from build123d import *

# Parameters (mm, degrees)
F1_DEPTH = 5
F2_R     = 1.5
F3_DEPTH = 25


with BuildPart() as f1:
    # F0 (on Front) → F1 (new body)
    with BuildSketch(Plane.XZ):
        with BuildLine():
            Line((-23, 75), (-27, 75))
            ThreePointArc((-27, 75), (-29.12132, 74.12132), (-30, 72))
            Line((-30, 72), (-30, -72))
            ThreePointArc((-30, -72), (-29.12132, -74.12132), (-27, -75))
            Line((-27, -75), (-23, -75))
            ThreePointArc((-23, -75), (-20.87868, -74.12132), (-20, -72))
            Line((-20, -72), (-20, -15))
            ThreePointArc((-20, -15), (-18.535534, -11.464466), (-15, -10))
            Line((-15, -10), (15, -10))
            ThreePointArc((15, -10), (18.535534, -11.464466), (20, -15))
            Line((20, -15), (20, -72))
            ThreePointArc((20, -72), (20.87868, -74.12132), (23, -75))
            Line((23, -75), (27, -75))
            ThreePointArc((27, -75), (29.12132, -74.12132), (30, -72))
            Line((30, -72), (30, 72))
            ThreePointArc((30, 72), (29.12132, 74.12132), (27, 75))
            Line((27, 75), (23, 75))
            ThreePointArc((23, 75), (20.87868, 74.12132), (20, 72))
            Line((20, 72), (20, 15))
            ThreePointArc((20, 15), (18.535534, 11.464466), (15, 10))
            Line((15, 10), (-15, 10))
            ThreePointArc((-15, 10), (-18.535534, 11.464466), (-20, 15))
            Line((-20, 15), (-20, 72))
            ThreePointArc((-20, 72), (-20.87868, 74.12132), (-23, 75))
        make_face()
        with BuildLine():
            Line((-23.600001, -71.399999), (-26.399999, -71.399999))
            Line((-26.399999, -71.399999), (-26.399999, 71.399999))
            Line((-26.399999, 71.399999), (-23.600001, 71.399999))
            Line((-23.600001, 71.399999), (-23.600001, 15))
            ThreePointArc((-23.600001, 15), (-21.081119, 8.918881), (-15, 6.399999))
            Line((-15, 6.399999), (15, 6.399999))
            ThreePointArc((15, 6.399999), (21.081119, 8.918881), (23.600001, 15))
            Line((23.600001, 15), (23.600001, 71.399999))
            Line((23.600001, 71.399999), (26.399999, 71.399999))
            Line((26.399999, 71.399999), (26.399999, -71.399999))
            Line((26.399999, -71.399999), (23.600001, -71.399999))
            Line((23.600001, -71.399999), (23.600001, -15))
            ThreePointArc((23.600001, -15), (21.081119, -8.918881), (15, -6.399999))
            Line((15, -6.399999), (-15, -6.399999))
            ThreePointArc((-15, -6.399999), (-21.081119, -8.918881), (-23.600001, -15))
            Line((-23.600001, -15), (-23.600001, -71.399999))
        make_face(mode=Mode.SUBTRACT)
    extrude(amount=F1_DEPTH)

    # F2 (on face) → F3 (cut)
    with BuildSketch(Plane.XY.offset(10)):
        with Locations((0, -2.50134)):
            Circle(F2_R)
    extrude(amount=-F3_DEPTH, mode=Mode.SUBTRACT)


solid = f1.part
CAD build for the part. Positions are in the model's coordinates, mm. A direction names the side the tool comes from. Coordinates: 2 decimals unless noted, no trailing zeros. Write each loop counter-clockwise with the first axis right and the second up, starting at its lowest first coordinate (ties: lowest second). Pieces come first, ordered by that corner, then holes. Notation, with made-up numbers: (87, 75) - (119, 75) arc R34 cw to (119, 111) - close; hole circle Ø2 at (47, 48). An arc over 180 degrees is marked (long way). Use a Markdown table: item, result. Add a question column.
Item 1: 3-axis set-ups, long thin cutter, end or side, ignore diameter. For faces 1 (the face through (20, -2, -43)), 2 (the face through (19, -2, 12)), 3 (the face through (25, -2, -71.4)), 4 (the face through (29.1, -2.46, -74.14)): which of +Z, -Z, +X, -X, +Y, -Y reach the whole face in a straight line?
Item 2: Drill centre lines: L1, parallel to X at y = -4.3, z = -35.5; L2, parallel to Z at x = 24.5, y = -0.8; L3, parallel to Z at x = -2, y = -0.65. Where is each one in solid material? Low to high. Write a range as from..to.
Item 3: Flat gauge pins, fed straight in: pin 1 (1.5 mm diameter, centred on x = 7, y = -3.5, fed in from +Z); pin 2 (1.8 mm diameter, centred on x = 0, y = -2.5, fed in from -Z). Where does each tip first touch, or does it go through?
Item 4: Mould opens along Y. For faces 5 (the face through (-25, -2, 71.4)), 6 (the face through (-20, 0, -11)), 7 (the face through (-1.5, -2.44, -8.17)) say: pulls with the +Y half, pulls with the -Y half, needs draft (parallel to the pull), parting line crosses it, or undercut.
Item 5: Band-saw the part on B-B, the plane z = -5. Give the cut face in (x, y).
Item 6: Band-saw the part on D-D, the plane z = -63. Give the cut face in (x, y), and give its area (3 significant figures).
Item 7: Band-saw the part on A-A, the plane x = 0. Give the cut face in (y, z), and give its area (3 significant figures).
Item 8: Band-saw the part on C-C, the plane x = -11. Give the cut face in (y, z), and give its area (3 significant figures).
Numbers:
| question | item | result |
|---|---|---|
| 1 | face 1 | -Z, +Y, -Y |
| 1 | face 2 | +Z, +Y, -Y |
| 1 | face 3 | +Y, -Y |
| 1 | face 4 | -Z, +X, +Y, -Y |
| 2 | L1 | -30..-26.4, -23.6..-20, 20..23.6, 26.4..30 |
| 2 | L2 | -75..-71.4, 71.4..75 |
| 2 | L3 | -10..-6.4, 6.4..10 |
| 3 | pin 1 | z = 10 |
| 3 | pin 2 | through |
| 4 | face 5 | needs draft |
| 4 | face 6 | pulls with the +Y half |
| 4 | face 7 | undercut |
| 5 | outline | (-30, -5) - (-26.4, -5) - (-26.4, 0) - (-30, 0) - close; (26.4, -5) - (30, -5) - (30, 0) - (26.4, 0) - close |
| 6 | outline | (-30, -5) - (-26.4, -5) - (-26.4, 0) - (-30, 0) - close; (-23.6, -5) - (-20, -5) - (-20, 0) - (-23.6, 0) - close; (20, -5) - (23.6, -5) - (23.6, 0) - (20, 0) - close; (26.4, -5) - (30, -5) - (30, 0) - (26.4, 0) - close |
| 6 | area | 72.0 mm2 |
| 7 | outline | (-5, -10) - (-4, -10) - (-4, -6.4) - (-5, -6.4) - close; (-5, 6.4) - (-4, 6.4) - (-4, 10) - (-5, 10) - close; (-1, -10) - (0, -10) - (0, -6.4) - (-1, -6.4) - close; (-1, 6.4) - (0, 6.4) - (0, 10) - (-1, 10) - close |
| 7 | area | 14.4 mm2 |
| 8 | outline | (-5, -10) - (0, -10) - (0, -6.4) - (-5, -6.4) - close; (-5, 6.4) - (0, 6.4) - (0, 10) - (-5, 10) - close |
| 8 | area | 36.0 mm2 |
